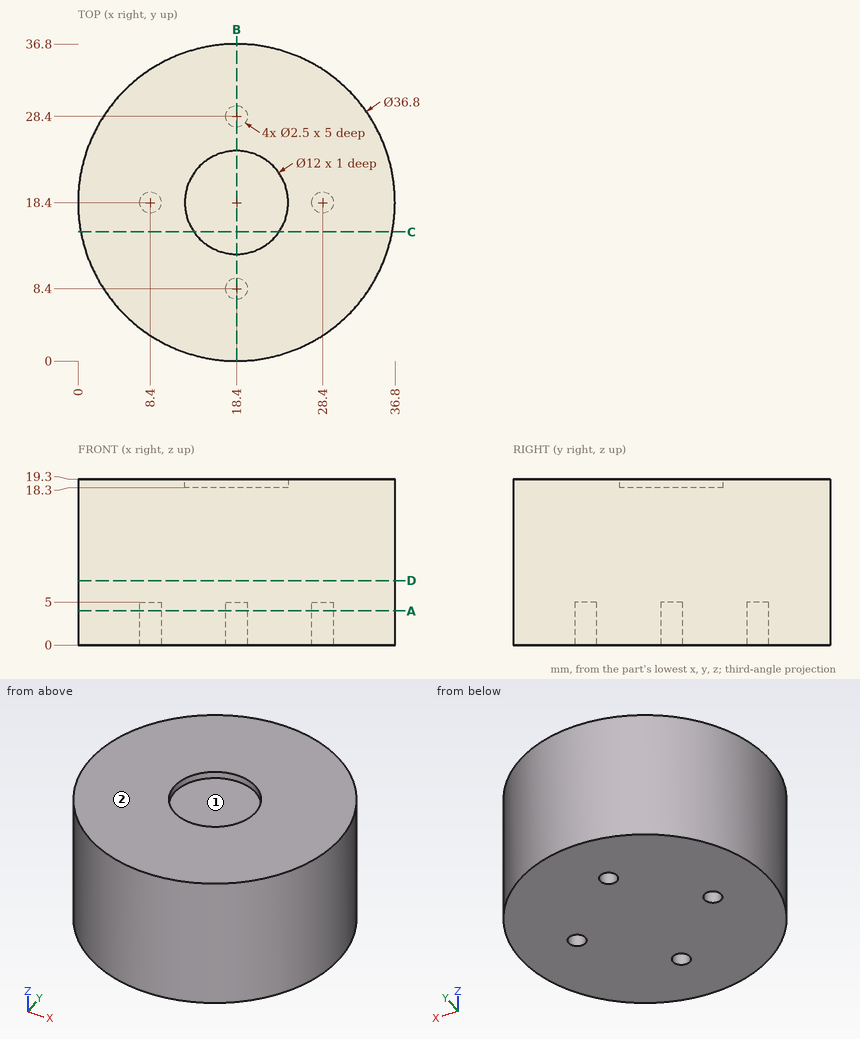
Verification items for this drawing (mm, ordinates from the low corner). A direction names the side the tool comes from. Give positions to 0.01 mm unless a question says otherwise; leave off trailing zeros. Loops run counter-clockwise (first coordinate to the right, second up) from the corner with the lowest first, then second, coordinate; pieces in that order, holes last. Notation, with made-up numbers: M 18,20 L 55,20 A18 ccw 55,31 Z; hole C 30.25,30 d5. An arc over 180 degrees is marked long. Answer as a JSON object with one key per item and string values. Group by question number.
Item 1: Sectioned sample at C-C on y = 15. Record the boundary of the cut face in (x, z).
Item 2: Sectioned sample at A-A on z = 4. Record the boundary of the cut face in (x, y).
Item 3: Material ranges on L1, parallel to Y at x = 18.4, z = 1.5; L2, parallel to Y at x = 18.4, z = 18.65; L3, parallel to X at y = 17.5, z = 4.5, recorded low to high.
Item 4: Sectioned sample at D-D on z = 7.5. Record the boundary of the cut face in (x, y), plus the area to 3 significant figures.
Item 5: Sectioned sample at B-B on x = 18.4. Record the boundary of the cut face in (y, z).
Item 6: Access from +Z, -Z, +X, -X, +Y, -Y to the whole of each face (thin tool, end or side, straight path). Record for the marked faces 1 and 2.
Item 7: Gauge pin test, flat ends, axial feed: pin 1 (1.5 mm diameter, centred on y = 12, z = 8.5, fed in from -X); pin 2 (6 mm diameter, centred on y = 29.5, z = 2.5, fed in from +X); pin 3 (6 mm diameter, centred on x = 19.5, z = 2.5, fed in from -Y); pin 4 (1.2 mm diameter, centred on x = 19, y = 8, fed in from -Z). Record the tip position at first contact, or that the pin passes through.
Findings below:
{
 "1": {"outline": "M 0.32,0 L 36.48,0 L 36.48,19.3 L 23.34,19.3 L 23.34,18.3 L 13.46,18.3 L 13.46,19.3 L 0.32,19.3 Z"},
 "2": {"outline": "C 18.4,18.4 d36.8; hole C 8.4,18.4 d2.5; hole C 18.4,8.4 d2.5; hole C 18.4,28.4 d2.5; hole C 28.4,18.4 d2.5"},
 "3": {"L1": "0 to 7.15, 9.65 to 27.15, 29.65 to 36.8", "L2": "0 to 12.4, 24.4 to 36.8", "L3": "0.02 to 7.53, 9.27 to 27.53, 29.27 to 36.78"},
 "4": {"outline": "C 18.4,18.4 d36.8", "area": "1,060 mm2"},
 "5": {"outline": "M 0,0 L 7.15,0 L 7.15,5 L 9.65,5 L 9.65,0 L 27.15,0 L 27.15,5 L 29.65,5 L 29.65,0 L 36.8,0 L 36.8,19.3 L 24.4,19.3 L 24.4,18.3 L 12.4,18.3 L 12.4,19.3 L 0,19.3 Z"},
 "6": {"face 1": "+Z", "face 2": "+Z, +X, -X, +Y, -Y"},
 "7": {"pin 1": "x = 0.89", "pin 2": "x = 34.92", "pin 3": "y = 0", "pin 4": "z = 0"}
}
